Design review of the part built by this model. Coordinates are the model's own, in mm. A direction names the side the tool comes from. Coordinates: 2 decimals unless noted, no trailing zeros. Write each loop counter-clockwise with the first axis right and the second up, starting at its lowest first coordinate (ties: lowest second). Pieces come first, ordered by that corner, then holes. Notation, with made-up numbers: (-35.75, 28.5) -> (-13.75, 28.5) arc R21 cw to (-13.75, 38.5) -> close; hole circle Ø10 at (-13.75, -26.75). An arc over 180 degrees is marked (long way). One line per question, with ' | ' between items. Start each with the question number.
Q1. For P1, Ø6, axis at x = 5, z = 5, coming from the -Y side, flat-tipped, find the tip position at first contact; note if it passes through.
Q2. Add section C-C on y = -0.5. State the section outline as (x, z) points, and give its area (3 significant figures).
Q3. Draft analysis for pull direction Z (two halves, no side actions). For faces 4 (the flat face through (0, 0, 0)), 5 (the cylindrical face through (1.97, -2.54, 8.3)), 6 (the flat face through (0, 0, 10)), 7 (the flat face through (0, -5, 5)), state which applies: pulls with the +Z half, pulls with the -Z half, needs draft (parallel to the pull), parting line crosses it, or undercut.
Q4. Wall thickness on probe 1 along Y at (x, z) = (-15, 6.7); probe 2 along X at (y, z) = (3.35, 5); probe 3 along X at (y, z) = (-3.25, 1.5): over which ranges is each line inside the solid? List them lowest first.
Q5. Add section B-B on x = -15. State the section outline as (y, z) points.
Q6. Add section A-A on z = 5. State the section outline as (x, y) points.
Q7. Add section D-D on y = 3.75. State the section outline as (x, z) points.
Q8. For faces 1 (the flat face through (-25, 0, 5)), 2 (the cylindrical face through (-0.627, -2.535, 5.971)), 3 (the cylindrical face through (17.5, 0.1, 2.1)), list the 3-axis set-ups (+Z, -Z, +X, -X, +Y, -Y) from which the entire face can be reached by the end or side of a thin tool; tool diameter is ignored.
from build123d import *

# Parameters (mm, degrees)
SKETCH1_W                               = 50
SKETCH1_H                               = 10
BOSS_EXTRUDE1_DEPTH                     = 10
CSK_FOR_M4_SFHCS1_AT_2_COUNT            = 2
CSK_FOR_M4_SFHCS1_AT_2_PITCH            = 10
CBORE_FOR_M5_HEX_HEAD_BOLT1_D           = 4.5
CBORE_FOR_M5_HEX_HEAD_BOLT1_CBORE_D     = 5
CBORE_FOR_M5_HEX_HEAD_BOLT1_CBORE_DEPTH = 4.2


with BuildPart() as part:
    # Sketch1 → Boss-Extrude1 (new body)
    with BuildSketch(Plane.XY):
        Rectangle(SKETCH1_W, SKETCH1_H)
    extrude(amount=BOSS_EXTRUDE1_DEPTH)

    # Sketch9 → CSK for M4 SFHCS1 (revolve, cut)
    with BuildSketch(Plane(origin=(5, -5, 5), x_dir=(0, 0, -1), z_dir=(1, 0, 0))):
        Polygon((0, 0), (0, 10), (2.25, 10), (2.25, 7.23), (4.48, 5), (4.48, 0), align=None)
    csk_for_m4_sfhcs1 = revolve(axis=Axis((5, -11.35, 5), (0, 1, 0)), mode=Mode.SUBTRACT)

    # CSK for M4 SFHCS1 at 2: CSK for M4 SFHCS1 ×2
    with Locations(*[(-i * CSK_FOR_M4_SFHCS1_AT_2_PITCH, 0, 0) for i in range(1, CSK_FOR_M4_SFHCS1_AT_2_COUNT)]):
        add(csk_for_m4_sfhcs1, mode=Mode.SUBTRACT)

    # CBORE for M5 Hex Head Bolt1 (through all)
    with Locations(Plane(origin=(0, 0, 0), x_dir=(-1, 0, 0), z_dir=(0, 0, -1))):
        with Locations((-15, 0), (15, 0)):
            CounterBoreHole(CBORE_FOR_M5_HEX_HEAD_BOLT1_D / 2, CBORE_FOR_M5_HEX_HEAD_BOLT1_CBORE_D / 2, CBORE_FOR_M5_HEX_HEAD_BOLT1_CBORE_DEPTH)


solid = part.part
Output values:
1) P1: stops at y = 1.48
2) outline: (-25, 0) -> (-17.45, 0) -> (-17.45, 4.2) -> (-17.19, 4.2) -> (-17.19, 10) -> (-25, 10) -> close; (-12.81, 4.2) -> (-12.55, 4.2) -> (-12.55, 0) -> (12.55, 0) -> (12.55, 4.2) -> (12.81, 4.2) -> (12.81, 10) -> (-12.81, 10) -> close; (17.19, 4.2) -> (17.45, 4.2) -> (17.45, 0) -> (25, 0) -> (25, 10) -> (17.19, 10) -> close; hole circle Ø8.96 at (-5, 5); hole circle Ø8.96 at (5, 5) | area: 282 mm2
3) face 4: pulls with the -Z half | face 5: undercut | face 6: pulls with the +Z half | face 7: needs draft
4) probe 1: y = -5 to -2.25, 2.25 to 5 | probe 2: x = -25 to -7.25, -2.75 to 2.75, 7.25 to 25 | probe 3: x = -25 to -7.8, -2.2 to 2.2, 7.8 to 25
5) outline: (-5, 0) -> (-2.5, 0) -> (-2.5, 4.2) -> (-2.25, 4.2) -> (-2.25, 10) -> (-5, 10) -> close; (2.25, 4.2) -> (2.5, 4.2) -> (2.5, 0) -> (5, 0) -> (5, 10) -> (2.25, 10) -> close
6) outline: (-25, -5) -> (-9.48, -5) -> (-9.48, 0) -> (-7.25, 2.23) -> (-7.25, 5) -> (-25, 5) -> close; (-2.75, 2.23) -> (-0.52, 0) -> (-0.52, -5) -> (0.52, -5) -> (0.52, 0) -> (2.75, 2.23) -> (2.75, 5) -> (-2.75, 5) -> close; (7.25, 2.23) -> (9.48, 0) -> (9.48, -5) -> (25, -5) -> (25, 5) -> (7.25, 5) -> close; hole circle Ø4.5 at (-15, 0); hole circle Ø4.5 at (15, 0)
7) outline: (-25, 0) -> (25, 0) -> (25, 10) -> (-25, 10) -> close; hole circle Ø4.5 at (-5, 5); hole circle Ø4.5 at (5, 5)
8) face 1: +Z, -Z, -X, +Y, -Y | face 2: -Y | face 3: -Z
